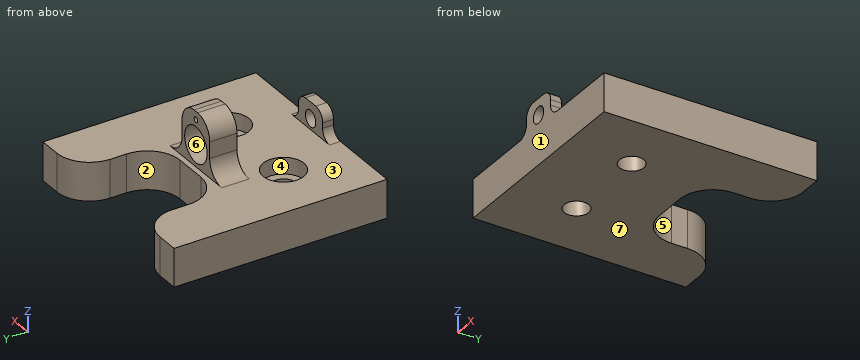
```python
from build123d import *

# Parameters (mm, degrees)
PAD_DEPTH       = 7
FILLET_R        = 6
SKETCH001_R     = 2.25
POCKET_DEPTH    = 8
SKETCH002_W     = 8
SKETCH002_H     = 5
PAD001_DEPTH    = 10
FILLET001_R     = 3.5
SKETCH003_R     = 3.25
SKETCH003_R_2   = 0.5
POCKET001_DEPTH = 7
SKETCH004_W     = 7
SKETCH004_H     = 2
PAD002_DEPTH    = 5
SKETCH005_R     = 1.5
POCKET002_DEPTH = 5
FILLET002_R     = 2
SKETCH006_R     = 3.75
POCKET003_DEPTH = 3


with BuildPart() as part:
    # Sketch → Pad (new body)
    with BuildSketch(Plane.XY):
        Polygon((19, 0), (-19, 0), (-19, 39), (-9, 39), (-9, 24), (9, 24), (9, 39), (19, 39), align=None)
    extrude(amount=PAD_DEPTH)

    # Fillet
    fillet_edges = [part.edges().sort_by_distance(p)[0] for p in [
        (-9, 39, 3.5),
        (-9, 24, 3.5),
        (9, 39, 3.5),
        (9, 24, 3.5),
    ]]
    fillet(fillet_edges, radius=FILLET_R)

    # Sketch001 (on Face5 of Fillet) → Pocket (cut)
    with BuildSketch(Plane.XY.offset(7)):
        with Locations((-8, 12)):
            Circle(SKETCH001_R)
        with Locations((8, 12)):
            Circle(SKETCH001_R)
    extrude(amount=-POCKET_DEPTH, mode=Mode.SUBTRACT)

    # Sketch002 (on Face5 of Pocket) → Pad001 (join)
    with BuildSketch(Plane.XY.offset(7)):
        with Locations((0, 20.5)):
            Rectangle(SKETCH002_W, SKETCH002_H)
    extrude(amount=PAD001_DEPTH)

    # Fillet001
    fillet001_edges = [part.edges().sort_by_distance(p)[0] for p in [
        (-4, 20.5, 7),
        (-4, 20.5, 17),
        (4, 20.5, 17),
        (4, 20.5, 7),
    ]]
    fillet(fillet001_edges, radius=FILLET001_R)

    # Sketch003 (on Face4 of Fillet001) → Pocket001 (cut)
    with BuildSketch(Plane.XZ.offset(-18)):
        with Locations((0, 11)):
            Circle(SKETCH003_R)
        with Locations((0, 15.5)):
            Circle(SKETCH003_R_2)
    extrude(amount=-POCKET001_DEPTH, mode=Mode.SUBTRACT)

    # Sketch004 (on Face1 of Pocket001) → Pad002 (join)
    with BuildSketch(Plane.XY.offset(7)):
        with Locations((0, 1)):
            Rectangle(SKETCH004_W, SKETCH004_H)
    extrude(amount=PAD002_DEPTH)

    # Sketch005 → Pocket002 (cut)
    with BuildSketch(Plane.XZ):
        with Locations((0, 9)):
            Circle(SKETCH005_R)
    extrude(amount=-POCKET002_DEPTH, mode=Mode.SUBTRACT)

    # Fillet002
    fillet002_edges = [part.edges().sort_by_distance(p)[0] for p in [
        (-3.5, 1, 12),
        (-3.5, 1, 7),
        (3.5, 1, 12),
        (3.5, 1, 7),
    ]]
    fillet(fillet002_edges, radius=FILLET002_R)

    # Sketch006 (on Face1 of Fillet002) → Pocket003 (cut)
    with BuildSketch(Plane.XY.offset(7)):
        with Locations((-8, 12)):
            Circle(SKETCH006_R)
        with Locations((8, 12)):
            Circle(SKETCH006_R)
    extrude(amount=-POCKET003_DEPTH, mode=Mode.SUBTRACT)


solid = part.part
```
For this review, take the finished solid that the model builds, in its own axes (mm). Face numbers are marked on the shaded views. A direction names the side the tool comes from. Give positions to 0.01 mm unless a question says otherwise; leave off trailing zeros. Order: outer loops, then holes, each group sorted by start corner. A loop starts at its lowest first (then second) coordinate and runs counter-clockwise, first axis right, second up.
1) The part is to be moulded in two halves that separate along Y. For the marked faces 1, 2, 3 and 4, say which applies: released by +Y, released by -Y, zero draft, split by the parting line, or undercut.
2) Insertion check: pin 1 (2 mm diameter, centred on x = -4, y = 5.5, fed in from +Z); pin 2 (0.6 mm diameter, centred on x = -0.5, y = 1.5, fed in from +Z); pin 3 (4 mm diameter, centred on x = -3, z = 14.5, fed in from -Y); pin 4 (1 mm diameter, centred on x = 6, z = 10, fed in from +Y). Each pin has a flat end and moves straight along its axis. Give the tip position at first contact, or say it passes through.
3) For the marked faces 5, 6 and 7, list the 3-axis set-ups (+Z, -Z, +X, -X, +Y, -Y) from which the entire face can be reached by the end or side of a thin tool; tool diameter is ignored.
4) Take a section at C-C (x = -2.5). Give the boundary of the cut face in (y, z).
5) Wall thickness on line 1 (Z direction, x = 0, y = 21.5); line 2 (Y direction, x = -3, z = 4); line 3 (Y direction, x = -1, z = 14.25): over which ranges is each line inside the solid? List them lowest first.
6) Take a section at B-B (z = 5.5). Give the boundary of the cut face in (x, y).
7) Take a section at A-A (y = 12). Give the boundary of the cut face in (x, z).
8) Take a section at D-D (y = 21.5). Give the boundary of the cut face in (x, z), then the cut area to 3 significant figures.
Derived:
1. face 1: released by -Y
1. face 2: released by +Y
1. face 3: undercut
1. face 4: undercut
2. pin 1: stops at z = 7
2. pin 2: stops at z = 12
2. pin 3: stops at y = 18
2. pin 4: passes through
3. face 5: +Z, -Z, +Y
3. face 6: +Y
3. face 7: -Z, +X, -X, +Y, -Y
4. outline: (0, 0) - (24, 0) - (24, 7) - (23, 7) - (23, 8.92) - (18, 8.92) - (18, 7) - (2, 7) - (2, 11.73) - (0, 11.73) - close; (18, 13.08) - (23, 13.08) - (23, 16.37) - (18, 16.37) - close
5. line 1: z = 0 to 7.75, 14.25 to 15, 16 to 17
5. line 2: y = 0 to 24
5. line 3: y = 18 to 23
6. outline: (-19, 0) - (19, 0) - (19, 39) - (15, 39) arc R6 ccw to (9, 33) - (9, 30) arc R6 cw to (3, 24) - (-3, 24) arc R6 cw to (-9, 30) - (-9, 33) arc R6 ccw to (-15, 39) - (-19, 39) - close; hole circle Ø7.5 at (-8, 12); hole circle Ø7.5 at (8, 12)
7. outline: (-19, 0) - (-10.25, 0) - (-10.25, 4) - (-11.75, 4) - (-11.75, 7) - (-19, 7) - close; (-5.75, 0) - (5.75, 0) - (5.75, 4) - (4.25, 4) - (4.25, 7) - (-4.25, 7) - (-4.25, 4) - (-5.75, 4) - close; (10.25, 0) - (19, 0) - (19, 7) - (11.75, 7) - (11.75, 4) - (10.25, 4) - close
8. outline: (-19, 0) - (19, 0) - (19, 7) - (7.5, 7) arc R3.5 cw to (4, 10.5) - (4, 13.5) arc R3.5 ccw to (0.5, 17) - (-0.5, 17) arc R3.5 ccw to (-4, 13.5) - (-4, 10.5) arc R3.5 cw to (-7.5, 7) - (-19, 7) - close; hole circle Ø6.5 at (0, 11); hole circle Ø1 at (0, 15.5)
8. area: 312 mm2
